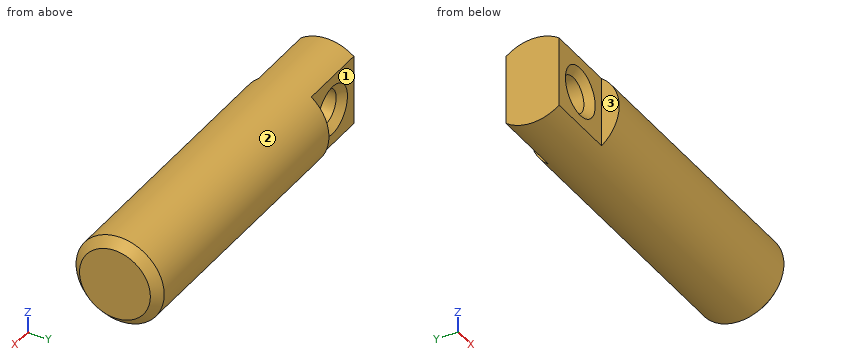
```python
from build123d import *

# Parameters (mm, degrees)
CUT_EXTRUDE1_DEPTH      = 2.5
CUT_EXTRUDE1_DEPTH_BACK = 2.5


with BuildPart() as part:
    # Sketch1 → Revolve1 (revolve)
    with BuildSketch(Plane.XY):
        Polygon((0, 0), (0, 2.5), (19.5095, 2.5), (20, 2.0095), (20, 0), align=None)
    revolve(axis=Axis((20, 0, 0), (-1, 0, 0)))

    # Sketch2 → Cut-Extrude1 (cut, two sides)
    with BuildSketch(Plane.XY) as cut_extrude1_sk:
        Polygon((-1, 3), (-1, -3), (4, -3), (4, -1.5), (0, -1.5), (0, 1.5), (4, 1.5), (4, 3), align=None)
    extrude(amount=CUT_EXTRUDE1_DEPTH, mode=Mode.SUBTRACT)
    extrude(cut_extrude1_sk.sketch, amount=-CUT_EXTRUDE1_DEPTH_BACK, mode=Mode.SUBTRACT)

    # Sketch3 → Cut-Revolve1 (revolve, cut)
    with BuildSketch(Plane.XY):
        Polygon((2, 1.5), (3.4, 1.5), (3, 1.1), (3, -1.1), (3.4, -1.5), (2, -1.5), align=None)
    revolve(axis=Axis((2, -1.5, 0), (0, 1, 0)), mode=Mode.SUBTRACT)


solid = part.part
```
Input: part model. Units: mm. Frame: model coordinates. Face numbers are marked on the shaded views. A direction names the side the tool comes from. Coordinates: 2 decimals unless noted, no trailing zeros. Loops run counter-clockwise (first coordinate to the right, second up) from the corner with the lowest first, then second, coordinate; pieces in that order, holes last. Notation, with made-up numbers: (17, -13) -> (46, -13) arc R22 ccw to (46, 11) -> close; hole circle Ø4 at (-0.75, -7). An arc over 180 degrees is marked (long way). Use a Markdown table: item, result.
1) Cut plane D-D (x = 17.5). Return the cut outline in (y, z).
Results found:
| item | result |
|---|---|
| outline | circle Ø5 at (0, 0) |
2) Access query for the marked faces 1, 2 and 3. Directions: +Z, -Z, +X, -X, +Y, -Y. A direction counts if a zero-diameter tool reaches every point of the face in a straight line with its end or side. Return the directions, or none.
Results found:
| item | result |
|---|---|
| face 1 | +Z, -Z, -X, +Y |
| face 2 | +X, -X |
| face 3 | +Z, -Z, -X, -Y |
3) Cut plane B-B (y = 0). Return the cut outline in (x, z), then the cut area to 3 significant figures.
Results found:
| item | result |
|---|---|
| outline | (0, -2.5) -> (19.51, -2.5) -> (20, -2.01) -> (20, 2.01) -> (19.51, 2.5) -> (0, 2.5) -> close; hole circle Ø2 at (2, 0) |
| area | 96.6 mm2 |
4) Cut plane C-C (x = 2). Return the cut outline in (y, z).
Results found:
| item | result |
|---|---|
| outline | (-1.5, -2) arc R2.5 ccw to (1.5, -2) -> (1.5, -1.4) -> (1.1, -1) -> (-1.1, -1) -> (-1.5, -1.4) -> close; (-1.5, 1.4) -> (-1.1, 1) -> (1.1, 1) -> (1.5, 1.4) -> (1.5, 2) arc R2.5 ccw to (-1.5, 2) -> close |
5) Contact query for flat-ended pins moving along their axis: pin 1 (3 mm diameter, centred on x = 8, y = -1.5, fed in from +Z); pin 2 (2 mm diameter, centred on x = 1.5, z = 0.5, fed in from +Y); pin 3 (1.5 mm diameter, centred on x = 10.5, y = 1, fed in from -Z); pin 4 (1.2 mm diameter, centred on x = 2, z = 0, fed in from -Y). Output: stop coordinate, or through.
Results found:
| item | result |
|---|---|
| pin 1 | stops at z = 2.5 |
| pin 2 | stops at y = 1.5 |
| pin 3 | stops at z = -2.49 |
| pin 4 | passes through |
6) Material intervals for line 1 along Z through (x, y) = (2, 0.1); line 2 along X through (y, z) = (0.1, 0); line 3 along Y through (x, z) = (7.5, 0.15), sorted ascending. Write a range as from..to.
Results found:
| item | result |
|---|---|
| line 1 | z = -2.5..-1, 1..2.5 |
| line 2 | x = 0..1, 3..20 |
| line 3 | y = -2.5..2.5 |
7) Cut plane A-A (z = 0). Return the cut outline in (x, y), then the cut area to 3 significant figures.
Results found:
| item | result |
|---|---|
| outline | (0, -1.5) -> (0.6, -1.5) -> (1, -1.1) -> (1, 1.1) -> (0.6, 1.5) -> (0, 1.5) -> close; (3, -1.1) -> (3.4, -1.5) -> (4, -1.5) -> (4, -2.5) -> (19.51, -2.5) -> (20, -2.01) -> (20, 2.01) -> (19.51, 2.5) -> (4, 2.5) -> (4, 1.5) -> (3.4, 1.5) -> (3, 1.1) -> close |
| area | 85.4 mm2 |
